```python
from build123d import *

# Parameters (mm, degrees)
EXTRUDE_1_DEPTH      = 2.1
EXTRUDE_1_DEPTH_BACK = 2.1
SKETCH_3_W           = 2.7
SKETCH_3_H           = 0.7
CUT_EXTRUDE_1_DEPTH  = 0.5
SKETCH_4_W           = 2.26
SKETCH_4_H           = 0.45
CUT_EXTRUDE_2_DEPTH  = 0.5
CHAMFER_1_SIZE       = 0.7
CUT_EXTRUDE_3_DEPTH  = 0.5
EXTRUDE_3_DEPTH      = 0.8
FILLET_1_R           = 0.2
FILLET_2_R           = 0.1
SKETCH_2_W           = 0.1
SKETCH_2_H           = 0.4
EXTRUDE_2_DEPTH      = 3


with BuildPart() as part:
    # Эскиз1 → Бобышка-Вытянуть1 (new, two sides: drawn at the far end of the back side and taken through both)
    with BuildSketch(Plane(origin=(0, 0, 0), x_dir=(1, 0, 0), z_dir=(0, 1, 0)).offset(-EXTRUDE_1_DEPTH_BACK)):
        Polygon((3.2, 0), (-3.2, 0), (-3.2, -5.4), (-1.5, -5.4), (-1.5, -1.5), (1.5, -1.5), (1.5, -5.4), (3.2, -5.4), align=None)
    extrude(amount=EXTRUDE_1_DEPTH + EXTRUDE_1_DEPTH_BACK)

    # Эскиз3 → Вырез-Вытянуть1 (cut)
    with BuildSketch(Plane(origin=(3.2, 0, 0), x_dir=(0, 0, -1), z_dir=(1, 0, 0))):
        with Locations((-4.05, 0)):
            Rectangle(SKETCH_3_W, SKETCH_3_H)
    cut_extrude_1 = extrude(amount=-CUT_EXTRUDE_1_DEPTH, mode=Mode.SUBTRACT)

    # Эскиз4 → Вырез-Вытянуть2 (cut)
    with BuildSketch(Plane.ZY.offset(-1.5)):
        with Locations((4.27, 0)):
            Rectangle(SKETCH_4_W, SKETCH_4_H)
    cut_extrude_2 = extrude(amount=-CUT_EXTRUDE_2_DEPTH, mode=Mode.SUBTRACT)

    # Зеркальное отражение1: Вырез-Вытянуть1, Вырез-Вытянуть2 across plane
    add(cut_extrude_1.mirror(Plane(origin=(0, 0, 0), x_dir=(0, 0, 1), z_dir=(1, 0, 0))), mode=Mode.SUBTRACT)
    add(cut_extrude_2.mirror(Plane(origin=(0, 0, 0), x_dir=(0, 0, 1), z_dir=(1, 0, 0))), mode=Mode.SUBTRACT)

    # Фаска1
    chamfer_1_edges = [part.edges().sort_by_distance(p)[0] for p in [
        (-2.35, -2.1, 5.4),
        (2.35, -2.1, 5.4),
    ]]
    chamfer(chamfer_1_edges, length=CHAMFER_1_SIZE)

    # Эскиз6 → Вырез-Вытянуть3 (cut)
    with BuildSketch(Plane(origin=(0, 0, 0), x_dir=(-1, 0, 0), z_dir=(0, 0, -1))):
        with BuildLine():
            Line((2.9, -1.6), (2.9, 1.6))
            Line((2.9, 1.6), (1.9, 1.6))
            Line((1.9, 1.6), (1.9, 0.8))
            Line((1.9, 0.8), (1.5, 0.8))
            Line((1.5, 0.8), (1.5, 1.6))
            Line((1.5, 1.6), (0.829156198, 1.6))
            ThreePointArc((0.829156198, 1.6), (0, 0.35), (-0.829156198, 1.6))
            Line((-0.829156198, 1.6), (-1.5, 1.6))
            Line((-1.5, 1.6), (-1.5, 0.8))
            Line((-1.5, 0.8), (-1.9, 0.8))
            Line((-1.9, 0.8), (-1.9, 1.6))
            Line((-1.9, 1.6), (-2.9, 1.6))
            Line((-2.9, 1.6), (-2.9, -1.6))
            Line((-2.9, -1.6), (-1.9, -1.6))
            Line((-1.9, -1.6), (-1.9, -0.8))
            Line((-1.9, -0.8), (-1.5, -0.8))
            Line((-1.5, -0.8), (-1.5, -1.6))
            Line((-1.5, -1.6), (-0.487339717, -1.6))
            ThreePointArc((-0.487339717, -1.6), (0, -0.65), (0.487339717, -1.6))
            Line((0.487339717, -1.6), (1.5, -1.6))
            Line((1.5, -1.6), (1.5, -0.8))
            Line((1.5, -0.8), (1.9, -0.8))
            Line((1.9, -0.8), (1.9, -1.6))
            Line((1.9, -1.6), (2.9, -1.6))
        make_face()
    extrude(amount=-CUT_EXTRUDE_3_DEPTH, mode=Mode.SUBTRACT)

    # Эскиз5 → Бобышка-Вытянуть3 (add)
    with BuildSketch(Plane(origin=(0, 0, 0), x_dir=(-1, 0, 0), z_dir=(0, 0, -1))):
        with BuildLine():
            Line((0.433012702, -1.5), (-0.433012702, -1.5))
            ThreePointArc((-0.433012702, -1.5), (0, -0.75), (0.433012702, -1.5))
        make_face()
        with BuildLine():
            Line((-0.683739717, 1.4), (0.683739717, 1.4))
            ThreePointArc((0.683739717, 1.4), (0, 0.55), (-0.683739717, 1.4))
        make_face()
    extrude(amount=EXTRUDE_3_DEPTH)

    # Скругление1
    fillet_1_edges = [part.edges().sort_by_distance(p)[0] for p in [
        (0, 0.55, -0.8),
        (0, 1.4, -0.8),
    ]]
    fillet(fillet_1_edges, radius=FILLET_1_R)

    # Скругление2
    fillet_2_edges = [part.edges().sort_by_distance(p)[0] for p in [
        (0, -0.75, -0.8),
        (0, -1.5, -0.8),
    ]]
    fillet(fillet_2_edges, radius=FILLET_2_R)

    # Эскиз2 → Бобышка-Вытянуть2 (add)
    with BuildSketch(Plane(origin=(0, 0, 0.5), x_dir=(-1, 0, 0), z_dir=(0, 0, -1))):
        with Locations((-2.5, 1.27)):
            Rectangle(SKETCH_2_W, SKETCH_2_H)
        with Locations((-2.5, -1.27)):
            Rectangle(SKETCH_2_W, SKETCH_2_H)
        with Locations((2.5, -1.27)):
            Rectangle(SKETCH_2_W, SKETCH_2_H)
        with Locations((2.5, 1.27)):
            Rectangle(SKETCH_2_W, SKETCH_2_H)
    extrude(amount=EXTRUDE_2_DEPTH)


solid = part.part
```
Input: part model. Units: mm. Frame: model coordinates. A direction names the side the tool comes from. Coordinates: 2 decimals unless noted, no trailing zeros. Order: outer loops, then holes, each group sorted by start corner. A loop starts at its lowest first (then second) coordinate and runs counter-clockwise, first axis right, second up. Notation, with made-up numbers: (59.5, -36) - (80.5, -36) arc R31 ccw to (80.5, -2) - close; hole circle Ø11 at (23, -21.75). An arc over 180 degrees is marked (long way). Put each result on its own line as item: value.
1. Line query: line 1 along X through (y, z) = (1.25, 2.5); line 2 along Z through (x, y) = (2.5, 1); line 3 along Z through (x, y) = (1.25, 0.9). Output: solid intervals per line, ascending.
Report:
line 1: x = -3.2 to -1.5, 1.5 to 3.2
line 2: z = 0.5 to 5.4
line 3: z = 0.5 to 1.5
2. Reachability of faces 1 (the face through (0, 0, 1.5)), 2 (the face through (2.3, 0.3, 5.4)), 3 (the face through (0, 0, 0.5)) from +Z, -Z, +X, -X, +Y, -Y: full face, straight path, thin tool, end or side. Return the list, or none.
Report:
face 1: +Z, +Y, -Y
face 2: +Z, +X, -X, +Y, -Y
face 3: -Z
3. Draft query along Y for faces 4 (the face through (-0.02, 0.55, -0.3)), 5 (the face through (-2.4, 0.3, 5.4)), 6 (the face through (0, -2.1, 1)). Return one class per face: pulls with the +Y half, pulls with the -Y half, needs draft (parallel to the pull), parting line crosses it, or undercut.
Report:
face 4: undercut
face 5: needs draft
face 6: pulls with the -Y half
4. Cut plane C-C on y = 1.75. Return the cut outline in (x, z).
Report:
outline: (-3.2, 0) - (3.2, 0) - (3.2, 5.4) - (1.5, 5.4) - (1.5, 1.5) - (-1.5, 1.5) - (-1.5, 5.4) - (-3.2, 5.4) - close
5. Cut plane B-B on z = -0.5. Return the cut outline in (x, y), then the cut area to 3 significant figures.
Report:
outline: (-2.55, -1.47) - (-2.45, -1.47) - (-2.45, -1.07) - (-2.55, -1.07) - close; (-2.55, 1.07) - (-2.45, 1.07) - (-2.45, 1.47) - (-2.55, 1.47) - close; (-0.68, 1.4) arc R0.7 ccw (long way) to (0.68, 1.4) - close; (-0.43, -1.5) - (0.43, -1.5) arc R0.5 ccw (long way) to start; (2.45, -1.47) - (2.55, -1.47) - (2.55, -1.07) - (2.45, -1.07) - close; (2.45, 1.07) - (2.55, 1.07) - (2.55, 1.47) - (2.45, 1.47) - close
area: 1.77 mm2
6. Cut plane D-D on x = 0. Return the cut outline in (y, z).
Report:
outline: (-2.1, 0) - (-1.5, 0) - (-1.5, -0.7) arc R0.1 ccw to (-1.4, -0.8) - (-0.85, -0.8) arc R0.1 ccw to (-0.75, -0.7) - (-0.75, 0) - (-0.65, 0) - (-0.65, 0.5) - (0.35, 0.5) - (0.35, 0) - (0.55, 0) - (0.55, -0.6) arc R0.2 ccw to (0.75, -0.8) - (1.2, -0.8) arc R0.2 ccw to (1.4, -0.6) - (1.4, 0) - (2.1, 0) - (2.1, 1.5) - (-2.1, 1.5) - close
7. Cut plane A-A on z = 2.5. Return the cut outline in (x, y), then the cut area to 3 significant figures.
Report:
outline: (-3.2, -2.1) - (-1.5, -2.1) - (-1.5, 2.1) - (-3.2, 2.1) - close; (1.5, -2.1) - (3.2, -2.1) - (3.2, 2.1) - (1.5, 2.1) - close
area: 14.3 mm2
